```python
from build123d import *

# Parameters (mm, degrees)
SKETCH1_R                               = 27
BOSS_EXTRUDE1_DEPTH                     = 5
BOSS_EXTRUDE3_DEPTH                     = 3
SKETCH2_3_R                             = 5
BOSS_EXTRUDE4_DEPTH                     = 5
CBORE_FOR_M5_HEX_HEAD_BOLT1_D           = 3
CBORE_FOR_M5_HEX_HEAD_BOLT1_CBORE_D     = 5
CBORE_FOR_M5_HEX_HEAD_BOLT1_CBORE_DEPTH = 1
SKETCH5_W                               = 39
SKETCH5_H                               = 30
CUT_EXTRUDE1_DEPTH                      = 1
SKETCH6_R                               = 1.5
CUT_EXTRUDE2_DEPTH                      = 42.910619179
CIRPATTERN1_COUNT                       = 4


with BuildPart() as part:
    # Sketch1 → Boss-Extrude1 (new body)
    with BuildSketch(Plane(origin=(0, 0, 0), x_dir=(1, 0, 0), z_dir=(0, 1, 0))):
        with Locations(Location((0, 0, 0), (0, 0, 270))):
            Circle(SKETCH1_R)
    extrude(amount=BOSS_EXTRUDE1_DEPTH)

    # Sketch2 → Boss-Extrude3 (add)
    with BuildSketch(Plane(origin=(0, 0, 0), x_dir=(1, 0, 0), z_dir=(0, 1, 0))):
        with BuildLine():
            ThreePointArc((-19.550252532, 23.792893219), (-20.964466094, 20.964466094), (-23.792893219, 19.550252532))
            Line((-23.792893219, 19.550252532), (-21.405668752, 16.455921283))
            ThreePointArc((-21.405668752, 16.455921283), (-19.091883092, 19.091883092), (-16.455921283, 21.405668752))
            Line((-16.455921283, 21.405668752), (-19.550252532, 23.792893219))
        make_face()
    boss_extrude3 = extrude(amount=BOSS_EXTRUDE3_DEPTH)

    # Sketch2<3> → Boss-Extrude4 (add, through all)
    with BuildSketch(Plane(origin=(0, 0, 0), x_dir=(1, 0, 0), z_dir=(0, 1, 0))):
        with Locations(Location((-24.5, 24.5, 0), (0, 0, 351.869897646))):
            Circle(SKETCH2_3_R)
    boss_extrude4 = extrude(amount=BOSS_EXTRUDE4_DEPTH)

    # CBORE for M5 Hex Head Bolt1 (through all)
    with Locations(Plane(origin=(0, 5, 0), x_dir=(1, 0, 0), z_dir=(0, 1, 0))):
        with Locations((-24.5, 24.5)):
            cbore_for_m5_hex_head_bolt1 = CounterBoreHole(CBORE_FOR_M5_HEX_HEAD_BOLT1_D / 2, CBORE_FOR_M5_HEX_HEAD_BOLT1_CBORE_D / 2, CBORE_FOR_M5_HEX_HEAD_BOLT1_CBORE_DEPTH)

    # Sketch5 → Cut-Extrude1 (cut)
    with BuildSketch(Plane(origin=(0, 5, 0), x_dir=(1, 0, 0), z_dir=(0, 1, 0))):
        Rectangle(SKETCH5_W, SKETCH5_H)
    extrude(amount=-CUT_EXTRUDE1_DEPTH, mode=Mode.SUBTRACT)

    # Sketch6 → Cut-Extrude2 (cut, through all)
    with BuildSketch(Plane(origin=(0, 4, 0), x_dir=(1, 0, 0), z_dir=(0, 1, 0))):
        with Locations(Location((-7.5, 0, 0), (0, 0, 270))):
            Circle(SKETCH6_R)
        with Locations(Location((7.5, 0, 0), (0, 0, 90))):
            Circle(SKETCH6_R)
    extrude(amount=-CUT_EXTRUDE2_DEPTH, mode=Mode.SUBTRACT)

    # CirPattern1: Boss-Extrude3, Boss-Extrude4, CBORE for M5 Hex Head Bolt1 ×4 about axis
    cirpattern1_axis = Axis((0, 0, 0), (0, 1, 0))
    add([boss_extrude3.rotate(cirpattern1_axis, i * 360 / CIRPATTERN1_COUNT) for i in range(1, CIRPATTERN1_COUNT)])
    add([boss_extrude4.rotate(cirpattern1_axis, i * 360 / CIRPATTERN1_COUNT) for i in range(1, CIRPATTERN1_COUNT)])
    add([cbore_for_m5_hex_head_bolt1.rotate(cirpattern1_axis, i * 360 / CIRPATTERN1_COUNT) for i in range(1, CIRPATTERN1_COUNT)], mode=Mode.SUBTRACT)


solid = part.part
```
Geometry: final body of the model. Coordinates: model frame, mm. A direction names the side the tool comes from. Round coordinates to 2 decimals unless told otherwise and drop trailing zeros. Loops run counter-clockwise (first coordinate to the right, second up) from the corner with the lowest first, then second, coordinate; pieces in that order, holes last. Notation, with made-up numbers: (-23.5, -24) -> (34.5, -24) arc R16 cw to (34.5, -3) -> close; hole circle Ø6 at (70.25, 44). An arc over 180 degrees is marked (long way). Use one line per item in the form item = value. Start each with the question number.
1) Draft query along Z for faces 1 (the cylindrical face through (27.67, 2.465, 28.366)), 2 (the flat face through (27, 5, -23)). Return one class per face: released by +Z, released by -Z, zero draft, split by the parting line, or undercut.
2) Section B-B on x = 24.5. Output: boundary loops of the cut face in (y, z).
3) First-contact query: P1, Ø3, axis at y = 4, z = -6.5, coming from the +X side; P2, Ø2.5, axis at x = -7.5, z = 0, coming from the -Y side; P3, Ø3, axis at y = 3.5, z = 4, coming from the -X side. Flat tips, straight axial feed; report the tip coordinate or a pass-through.
4) Section D-D on z = -13. Output: boundary loops of the cut face in (x, y).
5) Access query for faces 3 (the flat face through (20, 3, 20)), 4 (the flat face through (-27, 5, 23)). Directions: +Z, -Z, +X, -X, +Y, -Y. A direction counts if a zero-diameter tool reaches every point of the face in a straight line with its end or side. Return the directions, or none.
6) Section A-A on z = 0. Output: boundary loops of the cut face in (x, y).
7) Line query: L1, parallel to X at y = 1.75, z = 0; L2, parallel to Z at x = -24.5, y = 1.7; L3, parallel to Z at x = -24.5, y = 4.4. Output: solid intervals per line, ascending.
8) Section C-C on x = -7.5. Output: boundary loops of the cut face in (y, z).
Response:
q1.face_1 = undercut
q1.face_2 = zero draft
q2.outline = (0, -29.5) -> (5, -29.5) -> (5, -27) -> (4, -27) -> (4, -26) -> (0, -26) -> close; (0, -23) -> (4, -23) -> (4, -22) -> (5, -22) -> (5, -19.5) -> (0, -19.5) -> close; (0, -11.35) -> (5, -11.35) -> (5, 11.35) -> (0, 11.35) -> close; (0, 19.5) -> (5, 19.5) -> (5, 22) -> (4, 22) -> (4, 23) -> (0, 23) -> close; (0, 26) -> (4, 26) -> (4, 27) -> (5, 27) -> (5, 29.5) -> (0, 29.5) -> close
q3.P1 = 26.53
q3.P2 = through
q3.P3 = -26.88
q4.outline = (-23.66, 0) -> (23.66, 0) -> (23.66, 5) -> (19.5, 5) -> (19.5, 4) -> (-19.5, 4) -> (-19.5, 5) -> (-23.66, 5) -> close
q5.face_3 = +Y
q5.face_4 = +Z, -Z, +X, -X, +Y
q6.outline = (-27, 0) -> (-9, 0) -> (-9, 4) -> (-19.5, 4) -> (-19.5, 5) -> (-27, 5) -> close; (-6, 0) -> (6, 0) -> (6, 4) -> (-6, 4) -> close; (9, 0) -> (27, 0) -> (27, 5) -> (19.5, 5) -> (19.5, 4) -> (9, 4) -> close
q7.L1 = -27 to -9, -6 to 6, 9 to 27
q7.L2 = -29.5 to -26, -23 to -19.5, -11.35 to 11.35, 19.5 to 23, 26 to 29.5
q7.L3 = -29.5 to -27, -22 to -19.5, -11.35 to 11.35, 19.5 to 22, 27 to 29.5
q8.outline = (0, -25.94) -> (5, -25.94) -> (5, -15) -> (4, -15) -> (4, -1.5) -> (0, -1.5) -> close; (0, 1.5) -> (4, 1.5) -> (4, 15) -> (5, 15) -> (5, 25.94) -> (0, 25.94) -> close
